Autodesk Inventor part; units mm, degrees
ref_plane "YZ Plane" through (0, 0, 0) normal (1, 0, 0) x (0, 1, 0)
ref_plane "XZ Plane" through (0, 0, 0) normal (0, 1, 0) x (-1, 0, 0)
ref_plane "XY Plane" through (0, 0, 0) normal (0, 0, 1) x (1, 0, 0)
sketch "Sketch1" plane through (0, 0, 0) normal (0, 1, 0) x (-1, 0, 0)
  circle A0 centre (0, 0) radius 9.525
  circle A1 centre (0, 0) radius 6.985
  dimension "d0" = 19.05
  dimension "d1" = 2.54
  dimension "d2" = 13.97
extrude "Extrusion1" add sketch "Sketch1" along normal blind 711.2
sketch "Sketch3" plane through (0, 711.2, 0) normal (0, 1, 0) x (1, 0, 0)
  line L0 (12.7, -12.7) -> (-12.7, -12.7)
  line L1 (-12.7, -12.7) -> (-12.7, 12.7)
  line L2 (-12.7, 12.7) -> (12.7, 12.7)
  line L3 (12.7, 12.7) -> (12.7, -12.7)
  point P0 (0, 0)
  point P1 (0, 0)
  dimension "d7" = 25.4
  dimension "d8" = 25.4
extrude "Extrusion2" add sketch "Sketch3" along normal blind 25.4
sketch "Sketch4" plane through (12.7, 711.2, -12.7) normal (0, 0, -1) x (-1, 0, 0)
  line L0 (25.4, 0) -> (25.4, 25.4)
  line L1 (0, 0) -> (0, 25.4)
  circle A0 centre (12.7, 12.7) radius 6.35
  point P0 (12.7, -711.2)
  dimension "d11" = 12.7
extrude "Extrusion3" cut sketch "Sketch4" against normal blind 42.8625
properties part number "OuterLever"
Work out the finished part from the listing and answer in its coordinate system (mm). A direction names the side the tool comes from. Give positions to 0.01 mm unless a question says otherwise; leave off trailing zeros. Order: outer loops, then holes, each group sorted by start corner. A loop starts at its lowest first (then second) coordinate and runs counter-clockwise, first axis right, second up. Notation, with made-up numbers: (89.5, 37) -> (106.5, 37) arc R6 cw to (106.5, 41) -> close; hole circle Ø5 at (-14.75, 34.5). An arc over 180 degrees is marked (long way). Answer as a JSON object with one key per item and string values. Group by question number.
1. Section A-A on y = 723.9 is taken. Determine the outline of the cut face in (x, z), plus the area to 3 significant figures.
2. Flat-ended cylindrical pins translate along their axes: pin 1 Ø2 at (x, y) = (8, 498) entering from -Z; pin 2 Ø1 at (x, y) = (5, 448.5) entering from +Z (3 decimals); pin 3 Ø12 at (y, z) = (613.5, -2) entering from +X (3 decimals). Find the tip coordinate at first contact, or state that the pin passes through.
3. Section C-C on y = 554.5 is taken. Determine the outline of the cut face in (x, z) (3 decimals).
4. A tool of negligible diameter and unlimited length cuts with its end or side. For faces 5 (the cylindrical face through (7.559, 350.622, 5.796)), 6 (the flat face through (12.7, 724, 0)), from which of +Z, -Z, +X, -X, +Y, -Y can it reach the whole face along a straight path? Write none if from no direction.
5. Consider line 1 along Y through (x, z) = (0, -6.75); line 2 along Z through (x, y) = (0, 401) (3 decimals); line 3 along Y through (x, z) = (-1.25, -8.75). Determine where each line is inside the solid, lowest interval first. Write a range as [from, to].
6. The mould has two halves that part along Z. Classify faces 1 (the flat face through (-12.7, 724, 0)), 2 (the flat face through (0, 711.2, 0)), 3 (the flat face through (6, 721, 12.7)), 4 (the cylindrical face through (0.909, 350.622, -6.926)): released by +Z, released by -Z, zero draft, split by the parting line, or undercut.
7. Section B-B on x = 0 is taken. Determine the outline of the cut face in (y, z) (3 decimals), plus the area to 3 significant figures.
Result sheet:
{
 "1": {"outline": "(-12.7, -12.7) -> (-6.35, -12.7) -> (-6.35, 12.7) -> (-12.7, 12.7) -> close; (6.35, -12.7) -> (12.7, -12.7) -> (12.7, 12.7) -> (6.35, 12.7) -> close", "area": "323 mm^2"},
 "2": {"pin 1": "stops at z = -6.46", "pin 2": "stops at z = 8.395", "pin 3": "stops at x = 9.525"},
 "3": {"outline": "circle Ø19.05 at (0, 0); hole circle Ø13.97 at (0, 0)"},
 "4": {"face 5": "-Y", "face 6": "+Z, -Z, +X, +Y, -Y"},
 "5": {"line 1": "y = [711.2, 717.55], [730.25, 736.6]", "line 2": "z = [-9.525, -6.985], [6.985, 9.525]", "line 3": "y = [0, 717.67], [730.13, 736.6]"},
 "6": {"face 1": "zero draft", "face 2": "undercut", "face 3": "released by +Z", "face 4": "undercut"},
 "7": {"outline": "(0, -9.525) -> (711.2, -9.525) -> (711.2, -12.7) -> (717.55, -12.7) -> (717.55, 12.7) -> (711.2, 12.7) -> (711.2, 9.525) -> (0, 9.525) -> (0, 6.985) -> (711.2, 6.985) -> (711.2, -6.985) -> (0, -6.985) -> close; (730.25, -12.7) -> (736.6, -12.7) -> (736.6, 12.7) -> (730.25, 12.7) -> close", "area": "3,940 mm^2"}
}
